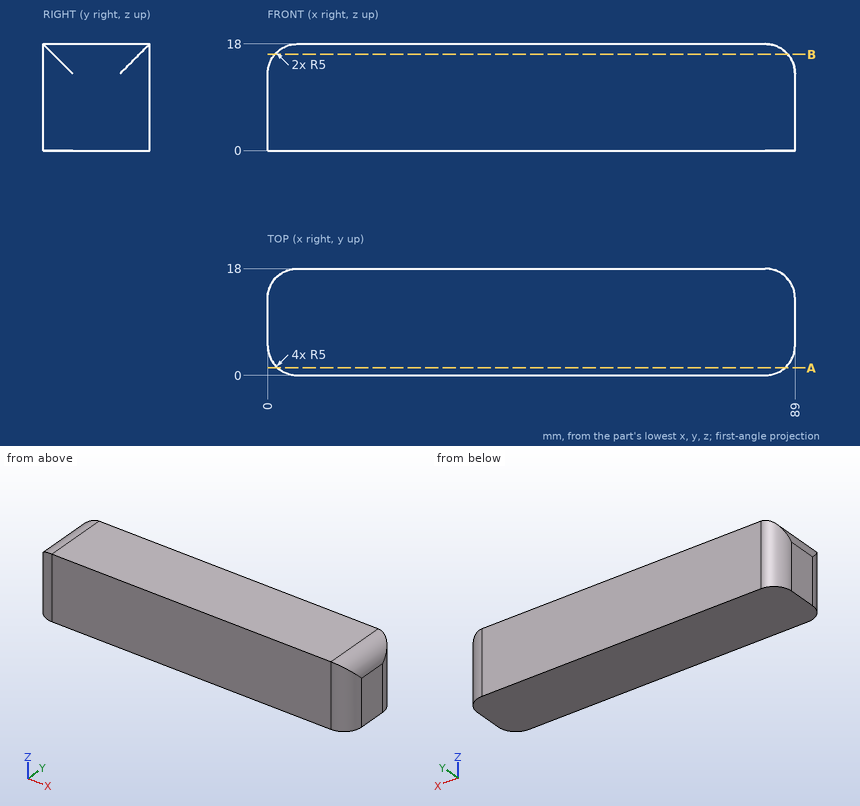
For this review, use the dimensioned drawing (mm, ordinates from the lowest corner) and the shaded views. Round coordinates to 2 decimals unless told otherwise and drop trailing zeros. Write each loop counter-clockwise with the first axis right and the second up, starting at its lowest first coordinate (ties: lowest second). Pieces come first, ordered by that corner, then holes. Notation, with made-up numbers: (66.5, 43) -> (86.5, 43) arc R36 cw to (86.5, 80) -> close; hole circle Ø1 at (1.25, 41.5). An arc over 180 degrees is marked (long way). Answer in a Markdown table with one row per item.
Q1. Take a section at B-B, the plane z = 16.25. State the section outline as (x, y) points, then the cut area to 3 significant figures.
The answers:
| item | result |
|---|---|
| outline | (1.2, 1.75) arc R5 ccw to (5, 0) -> (84, 0) arc R5 ccw to (87.8, 1.75) -> (87.8, 16.25) arc R5 ccw to (84, 18) -> (5, 18) arc R5 ccw to (1.2, 16.25) -> close |
| area | 1,550 mm² |
Q2. Take a section at A-A, the plane y = 1.25. State the section outline as (x, z) points.
The answers:
| item | result |
|---|---|
| outline | (1.69, 0) -> (87.31, 0) -> (87.31, 16.75) arc R5 ccw to (84, 18) -> (5, 18) arc R5 ccw to (1.69, 16.75) -> close |
Q3. To check wall thickness, follow L1, parallel to X at y = 1.75, z = 10.5; L2, parallel to X at y = 17.25, z = 5.75. State the ranges of each line that lie inside material, in increasing order. Write a range as [from, to].
The answers:
| item | result |
|---|---|
| L1 | [1.2, 87.8] |
| L2 | [2.37, 86.63] |
